Design review of the part built by this model. Coordinates are the model's own, in mm. A direction names the side the tool comes from. Round coordinates to 2 decimals unless told otherwise and drop trailing zeros. Loops run counter-clockwise (first coordinate to the right, second up) from the corner with the lowest first, then second, coordinate; pieces in that order, holes last. Notation, with made-up numbers: (-2, 14.5) -> (57, 14.5) arc R17 cw to (57, 20.5) -> close; hole circle Ø1 at (0, 49). An arc over 180 degrees is marked (long way). Use a Markdown table: item, result. Add a question column.
from build123d import *

# Parameters (mm, degrees)
BOSS_EXTRUDE1_DEPTH = 20
SKETCH2_W           = 15.981748592
SKETCH2_H           = 17.990874296
CUT_EXTRUDE1_DEPTH  = 15


with BuildPart() as part:
    # Sketch1 → Boss-Extrude1 (new body)
    with BuildSketch(Plane.XY):
        Polygon((0, 0), (0, 20), (35, 20), align=None)
    extrude(amount=BOSS_EXTRUDE1_DEPTH)

    # Sketch2 → Cut-Extrude1 (cut)
    with BuildSketch(Plane.ZY):
        with Locations((10.013945679, 8.995437148)):
            Rectangle(SKETCH2_W, SKETCH2_H)
    extrude(amount=-CUT_EXTRUDE1_DEPTH, mode=Mode.SUBTRACT)


solid = part.part
1. Insertion check: P1, Ø3, axis at y = 13.5, z = 8.5, coming from the -X side; P2, Ø1, axis at x = 11, z = 7.5, coming from the -Y side; P3, Ø8, axis at x = 19.5, z = 8, coming from the -Y side. Each pin has a flat end and moves straight along its axis. Give the tip position at first contact, or say it passes through.
2. To check wall thickness, follow probe 1 along Z at (x, y) = (9.5, 13.5); probe 2 along Y at (x, z) = (9.5, 14.75); probe 3 along X at (y, z) = (11, 17). State the ranges of each line that lie inside material, in increasing order. Write a range as from..to.
3. For faces 5 (the face through (7, 17.991, 10)), 6 (the face through (0, 19, 11)), list the 3-axis set-ups (+Z, -Z, +X, -X, +Y, -Y) from which the entire face can be reached by the end or side of a thin tool; tool diameter is ignored.
4. Consider section B-B on y = 7.75. State the section outline as (x, z) points, plus the area to 3 significant figures.
5. Consider section A-A on y = 15. State the section outline as (x, z) points.
6. Consider section C-C on x = 13. State the section outline as (y, z) points, plus the area to 3 significant figures.
7. Consider section D-D on z = 11. State the section outline as (x, y) points, plus the area to 3 significant figures.
8. Mouldability with a two-part tool opening along Z and no side actions: class faces 1 (the face through (10, 15, 0)), 2 (the face through (7, 11, 2.023)), 3 (the face through (17, 20, 10)), 4 (the face through (10, 15, 20)) as +Z half, -Z half, draft (parallel to the pull), parting line (faces both ways), or undercut.
Verdict:
| question | item | result |
|---|---|---|
| 1 | P1 | stops at x = 15 |
| 1 | P2 | stops at y = 17.99 |
| 1 | P3 | stops at y = 8.86 |
| 2 | probe 1 | z = 0..2.02, 18..20 |
| 2 | probe 2 | y = 17.99..20 |
| 2 | probe 3 | x = 15..19.25 |
| 3 | face 5 | -X, -Y |
| 3 | face 6 | +Z, -Z, -X, +Y, -Y |
| 4 | outline | (0, 0) -> (13.56, 0) -> (13.56, 2.02) -> (0, 2.02) -> close; (0, 18) -> (13.56, 18) -> (13.56, 20) -> (0, 20) -> close |
| 4 | area | 54.5 mm² |
| 5 | outline | (0, 0) -> (26.25, 0) -> (26.25, 20) -> (0, 20) -> (0, 18) -> (15, 18) -> (15, 2.02) -> (0, 2.02) -> close |
| 6 | outline | (7.43, 0) -> (20, 0) -> (20, 20) -> (7.43, 20) -> (7.43, 18) -> (17.99, 18) -> (17.99, 2.02) -> (7.43, 2.02) -> close |
| 6 | area | 82.6 mm² |
| 7 | outline | (0, 17.99) -> (15, 17.99) -> (15, 8.57) -> (35, 20) -> (0, 20) -> close |
| 7 | area | 144 mm² |
| 8 | face 1 | -Z half |
| 8 | face 2 | undercut |
| 8 | face 3 | draft |
| 8 | face 4 | +Z half |
